Could you check a few things on this model? Use its own coordinates, in mm. A direction names the side the tool comes from. Round coordinates to 2 decimals unless told otherwise and drop trailing zeros. Write each loop counter-clockwise with the first axis right and the second up, starting at its lowest first coordinate (ties: lowest second). Pieces come first, ordered by that corner, then holes. Notation, with made-up numbers: (32, -23.5) -> (87, -23.5) arc R24 cw to (87, -9.5) -> close; hole circle Ø8 at (61, 4). An arc over 180 degrees is marked (long way). Answer as CSV lines item,"result". Start each with the question number.
Q1. Will these pins go through, and if not, where does the flat tip stop? pin 1 Ø5 at (x, z) = (-21, 7) entering from +Y; pin 2 Ø9 at (y, z) = (-4.5, 7.5) entering from -X; pin 3 Ø4 at (y, z) = (-2, 2.5) entering from +X.
Q2. Imagine slicing it at C-C on x = -31.5. Please give me the cut outline in (y, z).
Q3. Imagine slicing it at B-B on z = 13. Please give me the cut outline in (x, y).
Q4. If we mould it in two halves opening along X, with no side actions, what happens to faces 6 (the cylindrical face through (-41.64, -13.07, 8.55)), 7 (the cylindrical face through (10.797, -12.93, 1.141)), 8 (the cylindrical face through (-31.12, -12.54, 14.18))? For each: pulls with the +X half, pulls with the -X half, needs draft (parallel to the pull), parting line crosses it, or undercut.
Q5. Imagine slicing it at A-A on y = -11.75. Give the number of separate pieces and of enclosed holes in the cut face, and give its area (3 significant figures).
Q6. If I drill on line 1 (X direction, y = -1.5, z = 8.75); line 2 (Y direction, x = -3.5, z = 4.5); line 3 (X direction, y = -12.25, z = 13.5), over which ranges is the centre line in solid material (lowest first)? Write a range as [from, to].
Q7. For faces 1 (the flat face through (-46, -8, 4)), 2 (the flat face through (-5, -6, 5)), 3 (the cylindrical face through (-39.2, -3.2, 1.5)), 4 (the flat face through (-5, -13, 12)), 5 (the flat face through (-0.99, -4.79, 7.14)), which set-ups out of +Z, -Z, +X, -X, +Y, -Y let a thin tool reach every point of the face, with its end or its side?
from build123d import *

# Parameters (mm, degrees)
BOSS_EXTRU_1_DEPTH           = 10
ESQUISSE2_W                  = 30.2
ESQUISSE2_H                  = 5
BOSS_EXTRU_2_DEPTH           = 9
ENL_V_MAT_EXTRU_1_DEPTH      = 47.925899032
ESQUISSE4_R                  = 1.6
ENL_V_MAT_EXTRU_2_DEPTH      = 47.925899032
ESQUISSE5_W                  = 30.2
ESQUISSE5_H                  = 2
ENL_V_MAT_EXTRU_3_DEPTH      = 47.925899032
CONG_2_R                     = 3
ESQUISSE6_W                  = 12
ESQUISSE6_H                  = 8
BOSS_EXTRU_3_DEPTH           = 10
ESQUISSE7_R                  = 1.7
ENL_V_MAT_EXTRU_4_DEPTH      = 58.773438571
CONG_3_R                     = 4
ENL_V_MAT_EXTRU_5_DEPTH      = 54.298876201
ENL_V_MAT_EXTRU_5_DEPTH_BACK = 54.298876201
ESQUISSE8_R                  = 1.7
ESQUISSE9_R                  = 3
ENL_V_MAT_EXTRU_6_DEPTH      = 2
ENL_V_MAT_EXTRU_7_DEPTH      = 2
CONG_4_R                     = 4
CONG_5_R                     = 4


# Some blends are built 0.0001 mm under size
with BuildPart() as part:
    # Esquisse1 → Boss.-Extru.1 (new body)
    with BuildSketch(Plane.XY):
        Polygon((-40.2, 0), (-35.2, 0), (-35.2, -10), (-5, -10), (-5, 0), (0, 0), (0, -18), (-40.2, -18), align=None)
    extrude(amount=BOSS_EXTRU_1_DEPTH)

    # Esquisse2 → Boss.-Extru.2 (add)
    with BuildSketch(Plane.XY.offset(10)):
        with Locations((-20.1, -12.5)):
            Rectangle(ESQUISSE2_W, ESQUISSE2_H)
    extrude(amount=BOSS_EXTRU_2_DEPTH)

    # Esquisse3 → Enlèv. mat.-Extru.1 (cut, through all)
    with BuildSketch(Plane.XZ.offset(15)):
        with BuildLine():
            Line((-31.2, 19), (-9, 19))
            ThreePointArc((-9, 19), (-20.1, 10), (-31.2, 19))
        make_face()
    extrude(amount=-ENL_V_MAT_EXTRU_1_DEPTH, mode=Mode.SUBTRACT)

    # Esquisse4 → Enlèv. mat.-Extru.2 (cut, through all)
    with BuildSketch(Plane.XZ.offset(15)):
        with Locations(Location((-32.2, 13, 0), (0, 0, 270))):
            Circle(ESQUISSE4_R)
        with Locations(Location((-8, 13, 0), (0, 0, 270))):
            Circle(ESQUISSE4_R)
    extrude(amount=-ENL_V_MAT_EXTRU_2_DEPTH, mode=Mode.SUBTRACT)

    # Esquisse5 → Enlèv. mat.-Extru.3 (cut, through all)
    with BuildSketch(Plane.XZ.offset(15)):
        with Locations((-20.1, 18)):
            Rectangle(ESQUISSE5_W, ESQUISSE5_H)
    extrude(amount=-ENL_V_MAT_EXTRU_3_DEPTH, mode=Mode.SUBTRACT)

    # Congé2
    # the kernel refuses this fillet: 3 mm, written as the material it takes off along each edge
    with BuildSketch(Plane(origin=(-5, -22.5, 17), x_dir=(0, 0, -1), z_dir=(0, 1, 0))) as cong_2_piece_1:
        with BuildLine():
            CenterArc((CONG_2_R, CONG_2_R), CONG_2_R, 180, 90)
            Line((0, CONG_2_R), (0, 0))
            Line((0, 0), (CONG_2_R, 0))
        make_face()
    extrude(amount=20, mode=Mode.SUBTRACT)
    with BuildSketch(Plane(origin=(-9.620019084, -5.395123123, 17), x_dir=(1, 0, 0), z_dir=(0, -1, 0))) as cong_2_piece_2:
        with BuildLine():
            CenterArc((1.841950751, -3), CONG_2_R, 90, 59.201185251)
            ThreePointArc((-0.734960717, -1.463924712), (-0.341024539, -0.745244452), (0, 0))
            Line((0, 0), (1.841950751, 0))
        make_face()
    extrude(amount=14.209753754, mode=Mode.SUBTRACT)
    with BuildSketch(Plane(origin=(-30.579980916, -5.395123123, 17), x_dir=(0.4486773426104955, 0, -0.8936938190610831), z_dir=(0, -1, 0))) as cong_2_piece_3:
        with BuildLine():
            CenterArc((1.854639889, -2.992172029), CONG_2_R, 94.139959503, 59.201185251)
            Line((-0.826441568, -1.646140001), (0, 0))
            ThreePointArc((0, 0), (0.819030344, -0.029602778), (1.638060688, 0))
        make_face()
    extrude(amount=14.209753754, mode=Mode.SUBTRACT)
    with BuildSketch(Plane(origin=(-35.2, -22.5, 17), x_dir=(0, 0, -1), z_dir=(0, 1, 0))) as cong_2_piece_4:
        with BuildLine():
            CenterArc((CONG_2_R, -CONG_2_R), CONG_2_R, 90, 90)
            Line((0, -CONG_2_R), (0, 0))
            Line((0, 0), (CONG_2_R, 0))
        make_face()
    extrude(amount=20, mode=Mode.SUBTRACT)

    # Esquisse6 → Boss.-Extru.3 (add)
    with BuildSketch(Plane.XZ.offset(18)):
        with Locations((-46.2, 4)):
            Rectangle(ESQUISSE6_W, ESQUISSE6_H)
        with Locations((6, 4)):
            Rectangle(ESQUISSE6_W, ESQUISSE6_H)
    extrude(amount=-BOSS_EXTRU_3_DEPTH)

    # Esquisse7 → Enlèv. mat.-Extru.4 (cut, through all)
    with BuildSketch(Plane.XZ.offset(18)):
        with Locations((-48.7, 4)):
            Circle(ESQUISSE7_R)
        with Locations((8.5, 4)):
            Circle(ESQUISSE7_R)
    extrude(amount=-ENL_V_MAT_EXTRU_4_DEPTH, mode=Mode.SUBTRACT)

    # Congé3
    cong_3_edges = [part.edges().sort_by_distance(p)[0] for p in [
        (-52.2, -13, 8),
        (-52.2, -13, 0),
        (12, -13, 0),
        (12, -13, 8),
    ]]
    fillet(cong_3_edges, radius=CONG_3_R - 0.0001)  # a hair under: the kernel refuses the full size

    # Esquisse8 → Enlèv. mat.-Extru.5 (cut, two sides: drawn at the far end of the back side and taken through both)
    with BuildSketch(Plane.ZY.offset(5).offset(-ENL_V_MAT_EXTRU_5_DEPTH_BACK)):
        with Locations((4.5, -3.3)):
            Circle(ESQUISSE8_R)
    extrude(amount=ENL_V_MAT_EXTRU_5_DEPTH + ENL_V_MAT_EXTRU_5_DEPTH_BACK, mode=Mode.SUBTRACT)

    # Esquisse9 → Enlèv. mat.-Extru.6 (cut)
    with BuildSketch(Plane.ZY.offset(40.2)):
        with Locations((4.5, -3.3)):
            Circle(ESQUISSE9_R)
    extrude(amount=-ENL_V_MAT_EXTRU_6_DEPTH, mode=Mode.SUBTRACT)

    # Esquisse10 → Enlèv. mat.-Extru.7 (cut)
    with BuildSketch(Plane(origin=(0, 0, 0), x_dir=(0, 0, -1), z_dir=(1, 0, 0))):
        Polygon((-8, -3.3), (-6.25, -6.331088913), (-2.75, -6.331088913), (-1, -3.3), (-2.75, -0.268911087), (-6.25, -0.268911087), align=None)
    extrude(amount=-ENL_V_MAT_EXTRU_7_DEPTH, mode=Mode.SUBTRACT)

    # Congé4
    cong_4_edges = [part.edges().sort_by_distance(p)[0] for p in [
        (-2.5, 0, 10),
        (-37.7, 0, 10),
    ]]
    fillet(cong_4_edges, radius=CONG_4_R)

    # Congé5
    # the kernel refuses this fillet: 4 mm, written as the material it adds along each edge
    with BuildSketch(Plane(origin=(0, -18, 8), x_dir=(0, 0, 1), z_dir=(0, 1, 0))) as cong_5_piece_1:
        with BuildLine():
            CenterArc((4, 3.464101615), CONG_5_R, 180, 60)
            Line((0, 3.464101615), (0, 0))
            Line((0, 0), (2, 0))
        make_face()
    extrude(amount=10)
    with BuildSketch(Plane(origin=(-40.2, -18, 8), x_dir=(0, 0, 1), z_dir=(0, 1, 0))) as cong_5_piece_2:
        with BuildLine():
            CenterArc((4, -3.464101615), CONG_5_R, 120, 60)
            Line((0, -3.464101615), (0, 0))
            Line((0, 0), (2, 0))
        make_face()
    extrude(amount=10)


solid = part.part
Checks:
1,pin 1,"y = -10"
1,pin 2,"x = -52.14"
1,pin 3,"x = 0"
2,outline,"(-18, 0) -> (-10, 0) -> (-10, 11.56) -> (-15, 11.56) -> (-15, 10) -> (-18, 10) -> close; (-15, 14.44) -> (-10, 14.44) -> (-10, 16.85) -> (-15, 16.85) -> close"
3,outline,"(-35.2, -15) -> (-33.8, -15) -> (-33.8, -10) -> (-35.2, -10) -> close; (-30.6, -15) -> (-27.79, -15) -> (-27.79, -10) -> (-30.6, -10) -> close; (-12.41, -15) -> (-9.6, -15) -> (-9.6, -10) -> (-12.41, -10) -> close; (-6.4, -15) -> (-5, -15) -> (-5, -10) -> (-6.4, -10) -> close"
4,face 6,"pulls with the -X half"
4,face 7,"pulls with the +X half"
4,face 8,"undercut"
5,separate pieces,"1"
5,enclosed holes,"4"
5,area,"650 mm^2"
6,line 1,"[-40.2, -35.2], [-5, 0]"
6,line 2,"[-18, -5], [-1.6, 0]"
6,line 3,"[-35.2, -33.72], [-30.68, -28.3], [-11.9, -9.52], [-6.48, -5]"
7,face 1,"+Z, -Z, -X, +Y"
7,face 2,"+Z, -Z, +Y"
7,face 3,"-X"
7,face 4,"+Z, +X, +Y, -Y"
7,face 5,"+X"
